from build123d import *
from OCP.BRepFilletAPI import BRepFilletAPI_MakeChamfer

# Parameters (mm, degrees)
FILLET2_R               = 0.5
FILLET3_R               = 0.3
SKETCH9_W               = 0.5
SKETCH9_H               = 1.95
BOSS_EXTRUDE5_DEPTH     = 3.6
CHAMFER2_SIZE           = 0.15
CHAMFER2_SIZE2          = 0.259807621
CUT_EXTRUDE2_DEPTH      = 25.309951666
CUT_EXTRUDE2_DEPTH_BACK = 25.309951666


with BuildPart() as part:
    # Sketch8 → Revolve1 (revolve)
    with BuildSketch(Plane(origin=(0, 0, 0), x_dir=(0, 0, -1), z_dir=(1, 0, 0)), mode=Mode.PRIVATE) as revolve1_sk:
        Polygon((0, 0), (0, 4.45), (2.2, 4.45), (2.2, 4.55), (1.7, 4.55), (1.7, 5), (3.2, 6.925), (3.4, 6.925), (3.4, 5.9), (12.45, 5.9), (12.85, 5.5), (16.95, 5.5), (16.95, 4.75), (18.65, 4.75), (18.65, 0), align=None)
    revolve(revolve1_sk.sketch.rotate(Axis((0, 0, 0), (0, 0, -1)), 90), axis=Axis((0, 0, 0), (0, 0, -1)))

    # Fillet2
    fillet2_edges = [part.edges().sort_by_distance(p)[0] for p in [
        (-5.5, 0, -16.95),
    ]]
    fillet(fillet2_edges, radius=FILLET2_R)

    # Fillet3
    fillet3_edges = [part.edges().sort_by_distance(p)[0] for p in [
        (-4.45, 0, 0),
    ]]
    fillet(fillet3_edges, radius=FILLET3_R)

    # Sketch9 → Boss-Extrude5 (add)
    with BuildSketch(Plane(origin=(0, 0, -18.65), x_dir=(-1, 0, 0), z_dir=(0, 0, -1))):
        with Locations((-3.7, 0)):
            Rectangle(SKETCH9_W, SKETCH9_H)
        with Locations((3.7, 0)):
            Rectangle(SKETCH9_W, SKETCH9_H)
    extrude(amount=BOSS_EXTRUDE5_DEPTH)

    # Chamfer2: one chamfer whose edges measure the first distance from different faces: ONE call of the kernel's chamfer builder (chamfer() names one face for all edges)
    chamfer2_edges_1 = [part.edges().sort_by_distance(p)[0] for p in [
        (3.45, 0, -22.25),
        (3.7, 0.975, -22.25),
        (3.95, 0, -22.25),
        (3.7, -0.975, -22.25),
    ]]
    chamfer2_side_1 = [part.faces().sort_by_distance(p)[0] for p in [
        (3.7, 0, -22.25),
    ]]
    chamfer2_edges_2 = [part.edges().sort_by_distance(p)[0] for p in [
        (-3.95, 0, -22.25),
        (-3.7, 0.975, -22.25),
        (-3.45, 0, -22.25),
        (-3.7, -0.975, -22.25),
    ]]
    chamfer2_side_2 = [part.faces().sort_by_distance(p)[0] for p in [
        (-3.7, 0, -22.25),
    ]]
    chamfer2 = BRepFilletAPI_MakeChamfer(part.part.solid().wrapped)
    for e in chamfer2_edges_1:
        chamfer2.Add(CHAMFER2_SIZE, CHAMFER2_SIZE2, e.wrapped, chamfer2_side_1[0].wrapped)  # the first distance lies on this face
    for e in chamfer2_edges_2:
        chamfer2.Add(CHAMFER2_SIZE, CHAMFER2_SIZE2, e.wrapped, chamfer2_side_2[0].wrapped)  # the first distance lies on this face
    add(Compound.cast(chamfer2.Shape()), mode=Mode.REPLACE)

    # Sketch10 → Cut-Extrude2 (cut, two sides: drawn at the far end of the back side and taken through both)
    with BuildSketch(Plane(origin=(0, 0, 0), x_dir=(0, 0, -1), z_dir=(1, 0, 0)).offset(-CUT_EXTRUDE2_DEPTH_BACK)):
        with BuildLine():
            Line((20.15, 0.45), (20.85, 0.45))
            ThreePointArc((20.85, 0.45), (21.3, 0), (20.85, -0.45))
            Line((20.85, -0.45), (20.15, -0.45))
            ThreePointArc((20.15, -0.45), (19.7, 0), (20.15, 0.45))
        make_face()
    extrude(amount=CUT_EXTRUDE2_DEPTH + CUT_EXTRUDE2_DEPTH_BACK, mode=Mode.SUBTRACT)


solid = part.part
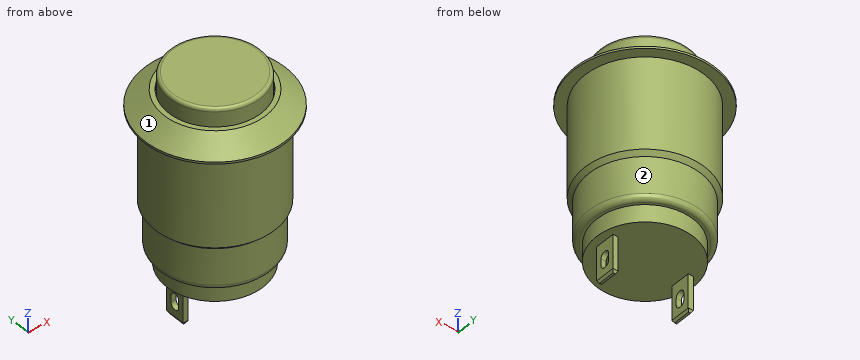
Design review of the part built by this model. Coordinates are the model's own, in mm. Face numbers are marked on the shaded views. A direction names the side the tool comes from. Coordinates: 2 decimals unless noted, no trailing zeros. Loops run counter-clockwise (first coordinate to the right, second up) from the corner with the lowest first, then second, coordinate; pieces in that order, holes last. Notation, with made-up numbers: M 75.5,18.5 L 132.5,18.5 A25 cw 132.5,34.5 Z; hole C 55.5,-1.75 d6. An arc over 180 degrees is marked long. Use one line per item in the form item = value.
(1) Clearance check with flat-ended pins moving along their axes: P1, Ø1, axis at x = -5, z = -9.5, coming from the -Y side; P2, Ø2, axis at y = 0, z = -20, coming from the -X side; P3, Ø2, axis at y = 0, z = -21, coming from the +X side. State where each tip first meets the part, or that it passes through.
Return value:
P1 = -3.82
P2 = -3.95
P3 = 3.95
(2) For line 1 along X through (y, z) = (-0.5, -20); line 2 along Z through (x, y) = (-0.75, -0.75); line 3 along X through (y, z) = (-3.5, -7), list the stretches that pass through material, from the lowest coordinate up. Write a range as from..to.
Return value:
line_1 = -3.95..-3.45, 3.45..3.95
line_2 = -18.65..0
line_3 = -4.75..4.75
(3) Consider section A-A (z = -20.5). Write out the cut boundary in (x, y) (3 decimals), and give its area (3 significant figures).
Return value:
outline = M -3.95,-0.975 L -3.45,-0.975 L -3.45,-0.45 L -3.95,-0.45 Z; M -3.95,0.45 L -3.45,0.45 L -3.45,0.975 L -3.95,0.975 Z; M 3.45,-0.975 L 3.95,-0.975 L 3.95,-0.45 L 3.45,-0.45 Z; M 3.45,0.45 L 3.95,0.45 L 3.95,0.975 L 3.45,0.975 Z
area = 1.05 mm2
(4) For the marked faces 1 and 2, list the 3-axis set-ups (+Z, -Z, +X, -X, +Y, -Y) from which the entire face can be reached by the end or side of a thin tool; tool diameter is ignored.
Return value:
face_1 = +Z
face_2 = -Z
(5) Consider section C-C (z = -13.25). Write out the cut boundary in (x, y).
Return value:
outline = C 0,0 d11
(6) Consider section D-D (z = -18.25). Write out the cut boundary in (x, y).
Return value:
outline = C 0,0 d9.5
